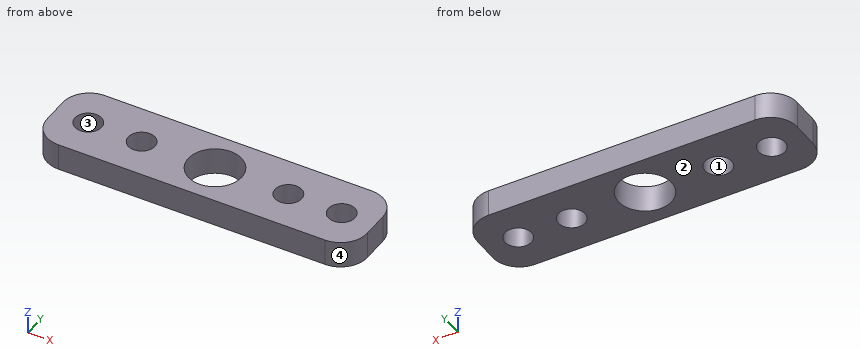
```python
from build123d import *

# Parameters (mm, degrees)
SKETCH1_R           = 2
SKETCH1_R_2         = 1
BOSS_EXTRUDE1_DEPTH = 2


with BuildPart() as part:
    # Sketch1 → Boss-Extrude1 (new body)
    with BuildSketch(Plane.XY):
        with BuildLine():
            Line((-4.75, 417.834574893), (15.25, 417.834574893))
            ThreePointArc((15.25, 417.834574893), (16.664213562, 417.248788455), (17.25, 415.834574893))
            Line((17.25, 415.834574893), (17.25, 413.834574893))
            ThreePointArc((17.25, 413.834574893), (16.664213562, 412.420361331), (15.25, 411.834574893))
            Line((15.25, 411.834574893), (-4.75, 411.834574893))
            ThreePointArc((-4.75, 411.834574893), (-6.164213562, 412.420361331), (-6.75, 413.834574893))
            Line((-6.75, 413.834574893), (-6.75, 415.834574893))
            ThreePointArc((-6.75, 415.834574893), (-6.164213562, 417.248788455), (-4.75, 417.834574893))
        make_face()
        with Locations((5.25, 414.834574893)):
            Circle(SKETCH1_R, mode=Mode.SUBTRACT)
        with Locations((10.75, 414.834574893)):
            Circle(SKETCH1_R_2, mode=Mode.SUBTRACT)
        with Locations((14.75, 414.834574893)):
            Circle(SKETCH1_R_2, mode=Mode.SUBTRACT)
        with Locations(Location((-0.25, 414.834574893, 0), (0, 0, 180))):
            Circle(SKETCH1_R_2, mode=Mode.SUBTRACT)
        with Locations(Location((-4.25, 414.834574893, 0), (0, 0, 180))):
            Circle(SKETCH1_R_2, mode=Mode.SUBTRACT)
    extrude(amount=BOSS_EXTRUDE1_DEPTH)


solid = part.part
```
Model file for the job. Use its own axes, mm. Face numbers are marked on the shaded views. Give positions to 0.01 mm unless a question says otherwise; leave off trailing zeros. Loops run counter-clockwise (first coordinate to the right, second up) from the corner with the lowest first, then second, coordinate; pieces in that order, holes last. Notation, with made-up numbers: (-2, -24.5) - (42, -24.5) arc R11 cw to (42, -18.5) - close; hole circle Ø2 at (65.5, 52). An arc over 180 degrees is marked (long way). One line per item, written item: value. Start each with the question number.
1. Slice it at D-D (x = 10.75). List the corners of the cut face in (y, z).
2. Slice it at B-B (y = 414.3). List the corners of the cut face in (x, z), plus the area to 3 significant figures.
3. Pull direction Y, two halves, no side cores. Call the marked faces 1, 2, 3 and 4: pulls with the +Y half, pulls with the -Y half, needs draft (parallel to the pull), parting line crosses it, or undercut.
4. Slice it at A-A (x = 5.25). List the corners of the cut face in (y, z).
5. Pin check, flat tip, straight feed: pin 1 (1.8 mm diameter, centred on x = 14.75, y = 414.83, fed in from +Z). Stop position of the tip, or through.
6. Probe L1, parallel to Y at x = 10.75, z = 1.55; L2, parallel to X at y = 414.9, z = 1.25; L3, parallel to X at y = 414.7, z = 1.8. List the from-to ranges inside material, lowest first. Write a range as from..to.
7. Slice it at C-C (z = 0.85). List the corners of the cut face in (x, y), plus the area to 3 significant figures.
Solution:
1. outline: (411.83, 0) - (413.83, 0) - (413.83, 2) - (411.83, 2) - close; (415.83, 0) - (417.83, 0) - (417.83, 2) - (415.83, 2) - close
2. outline: (-6.75, 0) - (-5.1, 0) - (-5.1, 2) - (-6.75, 2) - close; (-3.4, 0) - (-1.1, 0) - (-1.1, 2) - (-3.4, 2) - close; (0.6, 0) - (3.32, 0) - (3.32, 2) - (0.6, 2) - close; (7.18, 0) - (9.9, 0) - (9.9, 2) - (7.18, 2) - close; (11.6, 0) - (13.9, 0) - (13.9, 2) - (11.6, 2) - close; (15.6, 0) - (17.25, 0) - (17.25, 2) - (15.6, 2) - close
2. area: 26.8 mm^2
3. face 1: undercut
3. face 2: needs draft
3. face 3: undercut
3. face 4: pulls with the -Y half
4. outline: (411.83, 0) - (412.83, 0) - (412.83, 2) - (411.83, 2) - close; (416.83, 0) - (417.83, 0) - (417.83, 2) - (416.83, 2) - close
5. pin 1: passes through
6. L1: y = 411.83..413.83, 415.83..417.83
6. L2: x = -6.75..-5.25, -3.25..-1.25, 0.75..3.25, 7.25..9.75, 11.75..13.75, 15.75..17.25
6. L3: x = -6.75..-5.24, -3.26..-1.24, 0.74..3.25, 7.25..9.76, 11.74..13.76, 15.74..17.25
7. outline: (-6.75, 413.83) arc R2 ccw to (-4.75, 411.83) - (15.25, 411.83) arc R2 ccw to (17.25, 413.83) - (17.25, 415.83) arc R2 ccw to (15.25, 417.83) - (-4.75, 417.83) arc R2 ccw to (-6.75, 415.83) - close; hole circle Ø2 at (-4.25, 414.83); hole circle Ø2 at (-0.25, 414.83); hole circle Ø4 at (5.25, 414.83); hole circle Ø2 at (10.75, 414.83); hole circle Ø2 at (14.75, 414.83)
7. area: 115 mm^2
